Geometry: final body of the model. Coordinates: model frame, mm. Face numbers are marked on the shaded views. Coordinates: 2 decimals unless noted, no trailing zeros. Loops run counter-clockwise (first coordinate to the right, second up) from the corner with the lowest first, then second, coordinate; pieces in that order, holes last. Notation, with made-up numbers: (21.5, 42) - (76.5, 42) arc R11 ccw to (76.5, 50) - close; hole circle Ø3 at (51.25, -2.75). An arc over 180 degrees is marked (long way). Return JSON: item names as keys, results as strings.
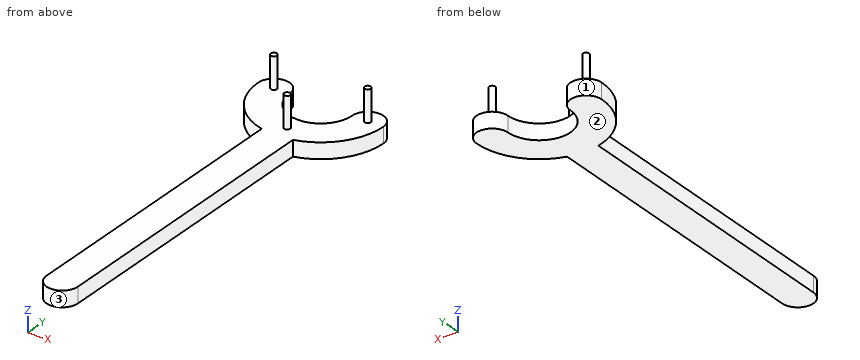
from build123d import *

# Parameters (mm, degrees)
BOX001_W          = 10
BOX001_H          = 100
BOX001_DEPTH      = 5
CYLINDER004_R     = 1
CYLINDER004_DEPTH = 10
CYLINDER005_R     = 1
CYLINDER005_DEPTH = 10
CYLINDER006_R     = 1
CYLINDER006_DEPTH = 10
CYLINDER007_R     = 5
CYLINDER007_DEPTH = 5
CYLINDER002_R     = 5
CYLINDER002_DEPTH = 5
CYLINDER003_R     = 5
CYLINDER003_DEPTH = 5
BOX_W             = 40
BOX_H             = 35
BOX_DEPTH         = 5
CYLINDER_R        = 10
CYLINDER_DEPTH    = 5
CYLINDER001_R     = 20
CYLINDER001_DEPTH = 5


with BuildPart() as cube001:
    # Box001 → Box001 (new body)
    with BuildSketch(Plane(origin=(-5, -115, 0), x_dir=(1, 0, 0), z_dir=(0, 0, 1))):
        with Locations((5, 50)):
            Rectangle(BOX001_W, BOX001_H)
    extrude(amount=BOX001_DEPTH)


with BuildPart() as cylinder004:
    # Cylinder004 → Cylinder004 (new body)
    with BuildSketch(Plane(origin=(0, -15, 5), x_dir=(1, 0, 0), z_dir=(0, 0, 1))):
        Circle(CYLINDER004_R)
    extrude(amount=CYLINDER004_DEPTH)


with BuildPart() as cylinder005:
    # Cylinder005 → Cylinder005 (new body)
    with BuildSketch(Plane(origin=(15, 0, 5), x_dir=(1, 0, 0), z_dir=(0, 0, 1))):
        Circle(CYLINDER005_R)
    extrude(amount=CYLINDER005_DEPTH)


with BuildPart() as cylinder006:
    # Cylinder006 → Cylinder006 (new body)
    with BuildSketch(Plane(origin=(-15, 0, 5), x_dir=(1, 0, 0), z_dir=(0, 0, 1))):
        Circle(CYLINDER006_R)
    extrude(amount=CYLINDER006_DEPTH)


with BuildPart() as cylinder007:
    # Cylinder007 → Cylinder007 (new body)
    with BuildSketch(Plane(origin=(0, -115, 0), x_dir=(1, 0, 0), z_dir=(0, 0, 1))):
        Circle(CYLINDER007_R)
    extrude(amount=CYLINDER007_DEPTH)


with BuildPart() as cylinder002:
    # Cylinder002 → Cylinder002 (new body)
    with BuildSketch(Plane(origin=(15, 0, 0), x_dir=(1, 0, 0), z_dir=(0, 0, 1))):
        Circle(CYLINDER002_R)
    extrude(amount=CYLINDER002_DEPTH)


with BuildPart() as cylinder003:
    # Cylinder003 → Cylinder003 (new body)
    with BuildSketch(Plane(origin=(-15, 0, 0), x_dir=(1, 0, 0), z_dir=(0, 0, 1))):
        Circle(CYLINDER003_R)
    extrude(amount=CYLINDER003_DEPTH)


with BuildPart() as cube:
    # Box → Box (new body)
    with BuildSketch(Plane(origin=(-20, 0, 0), x_dir=(1, 0, 0), z_dir=(0, 0, 1))):
        with Locations((20, 17.5)):
            Rectangle(BOX_W, BOX_H)
    extrude(amount=BOX_DEPTH)


with BuildPart() as cylinder:
    # Cylinder → Cylinder (new body)
    with BuildSketch(Plane.XY):
        Circle(CYLINDER_R)
    extrude(amount=CYLINDER_DEPTH)


with BuildPart() as obj1:
    # Cylinder001 → Cylinder001 (new body)
    with BuildSketch(Plane.XY):
        Circle(CYLINDER001_R)
    extrude(amount=CYLINDER001_DEPTH)

    # Cut: cut Cylinder
    add(cylinder.part, mode=Mode.SUBTRACT)

    # Cut001: cut Cube
    add(cube.part, mode=Mode.SUBTRACT)

    # Fusion: union Cylinder002, Cylinder003
    add(cylinder002.part)
    add(cylinder003.part)

    # Fusion001: union Cube001, Cylinder004, Cylinder005, Cylinder006, Cylinder007
    add(cube001.part)
    add(cylinder004.part)
    add(cylinder005.part)
    add(cylinder006.part)
    add(cylinder007.part)


solid = obj1.part
Item 1: Section query C-C, the plane y = -28. Return loops of the section in (x, z), and give its area (3 significant figures).
Worked out:
{"outline": "(-5, 0) - (5, 0) - (5, 5) - (-5, 5) - close", "area": "50.0 mm^2"}
Item 2: Mould query, pull axis X, two halves, no side actions, for the marked faces 1, 2 and 3. Classes: +X half, -X half, draft (parallel to the pull), parting line (faces both ways), or undercut.
Worked out:
{"face 1": "undercut", "face 2": "draft", "face 3": "parting line"}
Item 3: First-contact query: pin 1 Ø2.5 at (y, z) = (-86, 1.5) entering from -X; pin 2 Ø5 at (x, z) = (14, 3) entering from -Y; pin 3 Ø1.5 at (y, z) = (-71, 3.5) entering from +X. Flat tips, straight axial feed; report the tip coordinate or a pass-through.
Worked out:
{"pin 1": "x = -5", "pin 2": "y = -16.36", "pin 3": "x = 5"}
Item 4: Ray query, probe 1 along X at (y, z) = (-104, 2.5); probe 2 along Z at (x, y) = (1, -44); probe 3 along X at (y, z) = (0.5, 7.5). Return the intervals inside material, ascending. Write a range as from..to.
Worked out:
{"probe 1": "-5..5", "probe 2": "0..5", "probe 3": "-15.87..-14.13, 14.13..15.87"}
Item 5: Section query B-B, the plane z = 9. Return loops of the section in (x, y), and give its area (3 significant figures).
Worked out:
{"outline": "circle Ø2 at (-15, 0); circle Ø2 at (0, -15); circle Ø2 at (15, 0)", "area": "9.42 mm^2"}
Item 6: Section query A-A, the plane z = 2.25. Return loops of the section in (x, y).
Worked out:
{"outline": "(-20, 0) arc R20 ccw to (-5, -19.36) - (-5, -115) arc R5 ccw to (5, -115) - (5, -19.36) arc R20 ccw to (20, 0) arc R5 ccw to (10, 0) arc R10 cw to (-10, 0) arc R5 ccw to start"}
Item 7: Section query D-D, the plane x = -12.5. Return loops of the section in (y, z).
Worked out:
{"outline": "(-15.61, 0) - (4.33, 0) - (4.33, 5) - (-15.61, 5) - close"}
